Answer from the drawing. Dimensions are ordinates in mm from the lowest x, y and z of the part. A direction names the side the tool comes from. Round coordinates to 2 decimals unless told otherwise and drop trailing zeros. Write each loop counter-clockwise with the first axis right and the second up, starting at its lowest first coordinate (ties: lowest second). Pieces come first, ordered by that corner, then holes. Notation, with made-up numbers: (43.25, 55.25) - (65.25, 55.25) arc R16 ccw to (65.25, 82.25) - close; hole circle Ø6 at (57, 86). An arc over 180 degrees is marked (long way). One line per item, written item: value. Start each with the question number.
(1) For the marked faces 4, 5 and 6, determine the directions among +Z, -Z, +X, -X, +Y, -Y from which every point of the face is accessible in a straight line to the end or side of a thin tool.
(2) A cutting plane is placed at C-C, the plane z = 77.5. Determine the outline of the cut face in (x, y), plus the area to 3 significant figures.
(3) The mould has two halves that part along Z. Classify the marked faces 1, 2 and 3: +Z half, -Z half, draft (parallel to the pull), parting line (faces both ways), or undercut.
(4) Find the intervals of material crossed by L1, parallel to Z at x = 52, y = 5.75; L2, parallel to X at y = 2.25, z = 46.5; L3, parallel to Z at x = 48, y = 1.5, in increasing order.
(5) A cutting plane is placed at D-D, the plane x = 58. Determine the outline of the cut face in (y, z), plus the area to 3 significant figures.
(6) A cutting plane is placed at A-A, the plane y = 7.75. Determine the outline of the cut face in (x, z), plus the area to 3 significant figures.
(7) A cutting plane is placed at B-B, the plane x = 40. Determine the outline of the cut face in (y, z), plus the area to 3 significant figures.
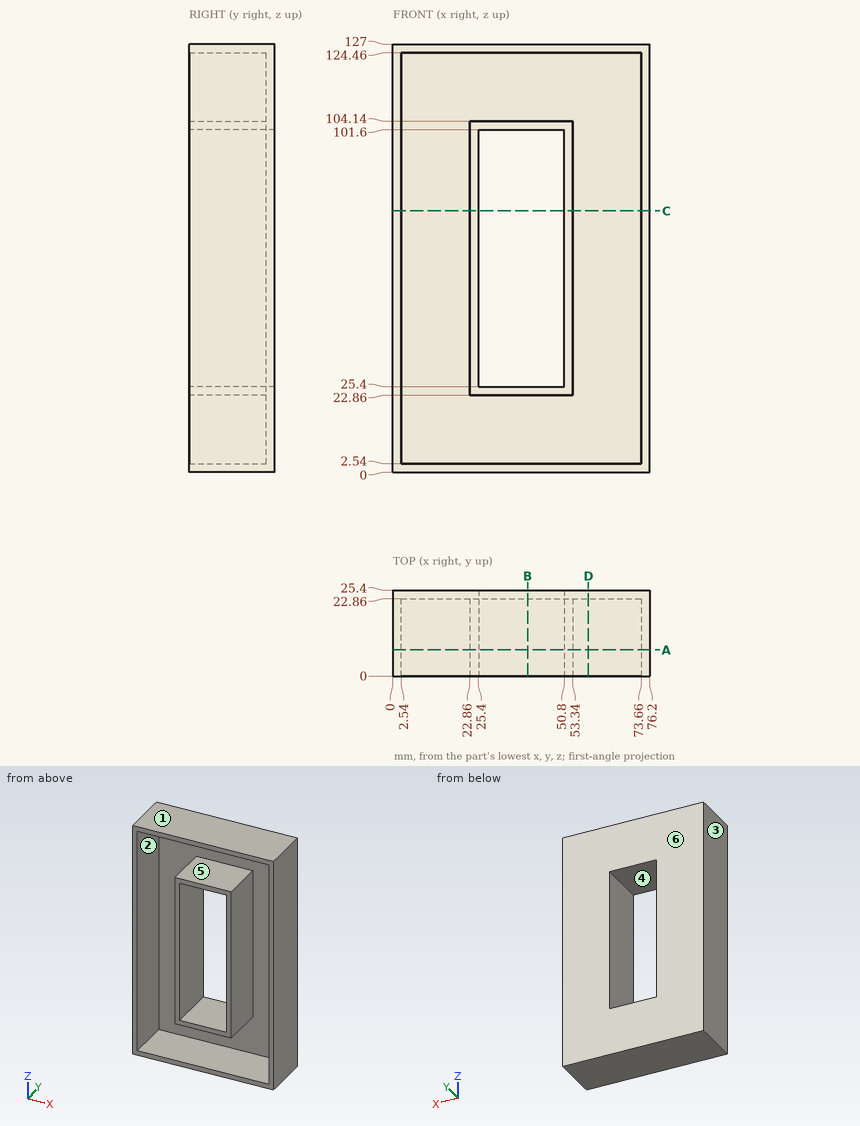
Here are the results:
1. face 4: +Y, -Y
1. face 5: -Y
1. face 6: +Z, -Z, +X, -X, +Y
2. outline: (0, 0) - (2.54, 0) - (2.54, 22.86) - (22.86, 22.86) - (22.86, 0) - (25.4, 0) - (25.4, 25.4) - (0, 25.4) - close; (50.8, 0) - (53.34, 0) - (53.34, 22.86) - (73.66, 22.86) - (73.66, 0) - (76.2, 0) - (76.2, 25.4) - (50.8, 25.4) - close
2. area: 361 mm²
3. face 1: +Z half
3. face 2: undercut
3. face 3: draft
4. L1: 0 to 2.54, 22.86 to 104.14, 124.46 to 127
4. L2: 0 to 2.54, 22.86 to 25.4, 50.8 to 53.34, 73.66 to 76.2
4. L3: 0 to 2.54, 22.86 to 25.4, 101.6 to 104.14, 124.46 to 127
5. outline: (0, 0) - (25.4, 0) - (25.4, 127) - (0, 127) - (0, 124.46) - (22.86, 124.46) - (22.86, 2.54) - (0, 2.54) - close
5. area: 439 mm²
6. outline: (0, 0) - (76.2, 0) - (76.2, 127) - (0, 127) - close; (22.86, 22.86) - (53.34, 22.86) - (53.34, 104.14) - (22.86, 104.14) - close; hole (2.54, 2.54) - (73.66, 2.54) - (73.66, 124.46) - (2.54, 124.46) - close; hole (25.4, 25.4) - (50.8, 25.4) - (50.8, 101.6) - (25.4, 101.6) - close
6. area: 1,550 mm²
7. outline: (0, 0) - (25.4, 0) - (25.4, 25.4) - (0, 25.4) - (0, 22.86) - (22.86, 22.86) - (22.86, 2.54) - (0, 2.54) - close; (0, 101.6) - (25.4, 101.6) - (25.4, 127) - (0, 127) - (0, 124.46) - (22.86, 124.46) - (22.86, 104.14) - (0, 104.14) - close
7. area: 361 mm²
